CAD build for the part. Positions are in the model's coordinates, mm. Give positions to 0.01 mm unless a question says otherwise; leave off trailing zeros. Write each loop counter-clockwise with the first axis right and the second up, starting at its lowest first coordinate (ties: lowest second). Pieces come first, ordered by that corner, then holes. Notation, with made-up numbers: (34.25, -36.75) - (80.25, -36.75) arc R36 ccw to (80.25, 0.25) - close; hole circle Ø4 at (79.5, 57). An arc over 180 degrees is marked (long way). Answer as a JSON object with one key per item and string values.
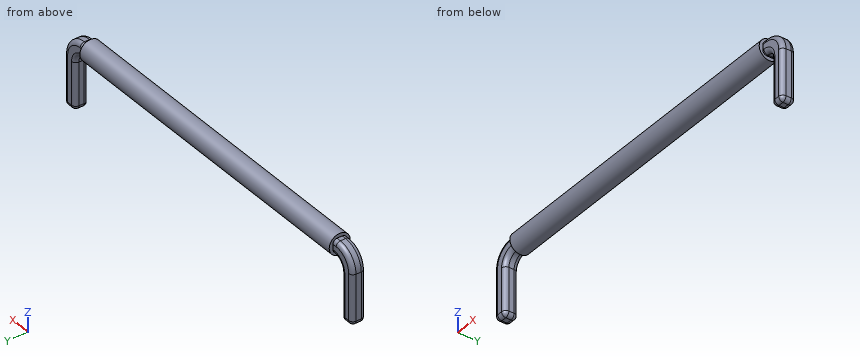
Autodesk Fusion 360 part; units mm, degrees
sketch "Sketch1" plane through (0, 0, 0) normal (1, 0, 0) x (0, 1, 0)
  circle A0 centre (0, 0) radius 0.5
  line L0 (0.325, -0.325) -> (-0.325, -0.325)
  line L1 (-0.325, -0.325) -> (-0.325, 0.325)
  line L2 (-0.325, 0.325) -> (0.325, 0.325)
  line L3 (0.325, 0.325) -> (0.325, -0.325)
  line L4 (0.325, -0.325) -> (-0.325, 0.325) construction
  line L5 (-0.325, -0.325) -> (0.325, 0.325) construction
  dimension "d1" = 1
  dimension "d2" = 0.65
  dimension "d3" = 0.65
extrude "Extrude1" add sketch "Sketch1" along normal blind 16 contours A0 | L0 L1 L2 L3
sketch "Sketch2" plane through (16, 0, 0) normal (1, 0, 0) x (0, 1, 0)
  circle A0 centre (0, 0) radius 0.5
  line L0 (0.325, -0.325) -> (-0.325, -0.325)
  line L1 (-0.325, -0.325) -> (-0.325, 0.325)
  line L2 (-0.325, 0.325) -> (0.325, 0.325)
  line L3 (0.325, 0.325) -> (0.325, -0.325)
  line L4 (0.325, -0.325) -> (-0.325, 0.325) construction
  line L5 (-0.325, -0.325) -> (0.325, 0.325) construction
  dimension "d8" = 0.65
  dimension "d9" = 0.65
extrude "Extrude2" add sketch "Sketch2" along normal blind 1.215 contours L0 L1 L2 L3
extrude "Extrude3" add sketch "Sketch1" against normal blind 1.215 contours L0 L1 L2 L3
sketch "Sketch3" plane through (0, 0, -0.325) normal (0, 0, -1) x (1, 0, 0)
  line L0 (16, 0.325) -> (16, -0.325)
  line L1 (16, -0.325) -> (17.215, -0.325)
  line L2 (17.215, -0.325) -> (17.215, 0.325)
  line L3 (17.215, 0.325) -> (16, 0.325)
  line L4 (17.215, 0.325) -> (16.565, 0.325)
  line L5 (16.565, 0.325) -> (16.565, -0.325)
  line L6 (16.565, -0.325) -> (17.215, -0.325)
  line L7 (17.215, -0.325) -> (17.215, 0.325)
  line L8 (17.215, 0.325) -> (16.565, -0.325) construction
  line L9 (16.565, 0.325) -> (17.215, -0.325) construction
  point P0 (16.89, 0)
  dimension "d14" = 0.65
  dimension "d15" = 0.65
sketch "Sketch4" plane through (0, 0, -0.325) normal (0, 0, -1) x (1, 0, 0)
  line L0 (0, -0.325) -> (0, 0.325)
  line L1 (0, 0.325) -> (-1.215, 0.325)
  line L2 (-1.215, 0.325) -> (-1.215, -0.325)
  line L3 (-1.215, -0.325) -> (0, -0.325)
  line L4 (-0.565, -0.325) -> (-1.215, -0.325)
  line L5 (-1.215, -0.325) -> (-1.215, 0.325)
  line L6 (-1.215, 0.325) -> (-0.565, 0.325)
  line L7 (-0.565, 0.325) -> (-0.565, -0.325)
  line L8 (-0.565, -0.325) -> (-1.215, 0.325) construction
  line L9 (-1.215, -0.325) -> (-0.565, 0.325) construction
  point P0 (-0.89, 0)
  dimension "d17" = 0.65
  dimension "d18" = 0.65
extrude "Extrude4" add sketch "Sketch4" sketch "Sketch3" along normal blind 2.75 contours L1 L2 L3 L4 L5 L6 L7 of sketch 2 contours L1 L2 L3 L4 L5 L6 L7
fillet "Fillet1" radius 0.5 2 edges at (-0.565, 0, -0.325) (16.565, 0, -0.325)
fillet "Fillet2" radius 1 2 edges at (-1.215, 0, 0.325) (17.215, 0, 0.325)
fillet "Fillet3" radius 0.2 28 edges at (-0.89, -0.325, -3.075) (-0.565, 0, -3.075) (-0.89, 0.325, -3.075) (-1.215, 0, -3.075) (-0.4186, -0.325, -0.4714) (-0.565, -0.325, -1.95) (-0.1075, -0.325, 0.325) (-0.9221, -0.325, 0.0321) (-1.215, -0.325, -1.875) (-0.1075, 0.325, 0.325) (-0.9221, 0.325, 0.0321) (-1.215, 0.325, -1.875) (-0.4186, 0.325, -0.4714) (-0.565, 0.325, -1.95) (16.1075, -0.325, 0.325) (16.9221, -0.325, 0.0321) (17.215, -0.325, -1.875) (16.565, -0.325, -1.95) (16.4186, -0.325, -0.4714) (17.215, 0.325, -1.875) (16.9221, 0.325, 0.0321) (16.1075, 0.325, 0.325) (16.4186, 0.325, -0.4714) (16.565, 0.325, -1.95) (16.89, 0.325, -3.075) (17.215, 0, -3.075) (16.89, -0.325, -3.075) (16.565, 0, -3.075)
equation "d1 = width"
equation "d2 = d3"
equation "d3 = d1 * 0.65"
equation "width = 1 mm"
equation "baseLenght = 16 mm"
equation "d6 = baseLenght"
equation "d8 = width * 0.65"
equation "d9 = d8"
equation "d14 = width * 0.65"
equation "d15 = d14"
equation "d17 = width * 0.65"
equation "d18 = d17"
equation "d26 = 0.2 * width"
(1) Saw through at A-A, the plane z = -1.7. Give the cut face in (x, y) (3 decimals), and give its area (3 significant figures).
Answer key:
{"outline": "(-1.215, -0.125) arc R0.2 ccw to (-1.015, -0.325) - (-0.765, -0.325) arc R0.2 ccw to (-0.565, -0.125) - (-0.565, 0.125) arc R0.2 ccw to (-0.765, 0.325) - (-1.015, 0.325) arc R0.2 ccw to (-1.215, 0.125) - close; (16.565, -0.125) arc R0.2 ccw to (16.765, -0.325) - (17.015, -0.325) arc R0.2 ccw to (17.215, -0.125) - (17.215, 0.125) arc R0.2 ccw to (17.015, 0.325) - (16.765, 0.325) arc R0.2 ccw to (16.565, 0.125) - close", "area": "0.776 mm²"}
(2) Flat gauge pins, fed straight in: P1, Ø1.1, axis at x = -1, z = -2, coming from the -Y side (3 decimals); P2, Ø0.8, axis at x = -0.5, z = -1.5, coming from the +Y side (3 decimals); P3, Ø0.5, axis at y = 0, z = 0, coming from the -X side. Where does each tip first touch, or does it go through?
Answer key:
{"P1": "stops at y = -0.325", "P2": "stops at y = 0.325", "P3": "stops at x = -1.12"}
(3) Saw through at B-B, the plane x = 2. Give the cut face in (y, z).
Answer key:
{"outline": "circle Ø1 at (0, 0)"}
(4) Probe L1, parallel to X at y = 0.15, z = -1.05; L2, parallel to Z at x = 9.25, y = -0.05; L3, parallel to Z at x = 1.25, y = 0.35. List the from-to ranges inside material, lowest first. Write a range as [from, to].
Answer key:
{"L1": "x = [-1.21, -0.57], [16.57, 17.21]", "L2": "z = [-0.5, 0.5]", "L3": "z = [-0.36, 0.36]"}
